Read the model definition and answer for the solid it produces. Units are mm, in the model's axes. Face numbers are marked on the shaded views. A direction names the side the tool comes from. Round coordinates to 2 decimals unless told otherwise and drop trailing zeros. Loops run counter-clockwise (first coordinate to the right, second up) from the corner with the lowest first, then second, coordinate; pieces in that order, holes last. Notation, with made-up numbers: M 52,84 L 72,84 A26 ccw 72,109 Z; hole C 48,37 d3. An arc over 180 degrees is marked long. Answer as CSV lines item,"result".
```python
from build123d import *

# Parameters (mm, degrees)
F0_W     = 48
F0_H     = 11
F1_DEPTH = 1.1
F0_W_2   = 52
F0_H_2   = 14
F2_DEPTH = 6
F3_R     = 0.925956
F4_DEPTH = 25


with BuildPart() as f1:
    # F0 (on Top) → F1 (new body)
    with BuildSketch(Plane.XY):
        Rectangle(F0_W, F0_H)
    extrude(amount=F1_DEPTH)

    # F0 (on Top) → F2 (join)
    with BuildSketch(Plane.XY):
        Rectangle(F0_W_2, F0_H_2)
        Rectangle(F0_W, F0_H, mode=Mode.SUBTRACT)
    extrude(amount=F2_DEPTH)

    # F3 (on face) → F4 (cut)
    with BuildSketch(Plane(origin=(24, 0, 0), x_dir=(0, -1, 0), z_dir=(-1, 0, 0))):
        with Locations((0, 3.55)):
            Circle(F3_R)
    extrude(amount=-F4_DEPTH, mode=Mode.SUBTRACT)


solid = f1.part
```
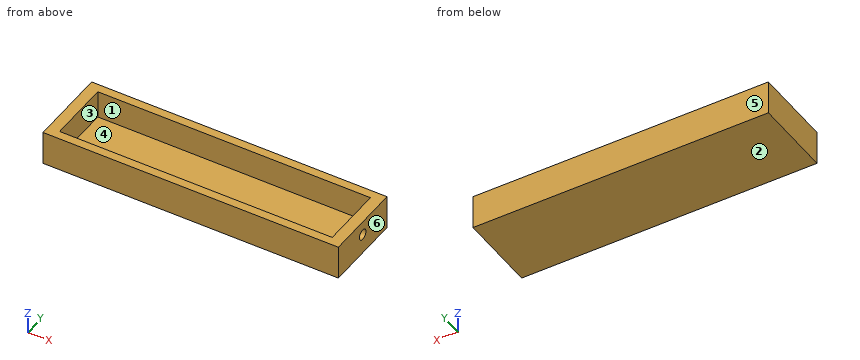
1) Find section D-D, the plane y = 0. Give the vertices of the cut face in (x, z).
Evaluation:
outline,"M -26,0 L 26,0 L 26,2.62 L 24,2.62 L 24,1.1 L -24,1.1 L -24,6 L -26,6 Z; M 24,4.48 L 26,4.48 L 26,6 L 24,6 Z"
2) Find section C-C, the plane x = 21. Give the vertices of the cut face in (y, z).
Evaluation:
outline,"M -7,0 L 7,0 L 7,6 L 5.5,6 L 5.5,1.1 L -5.5,1.1 L -5.5,6 L -7,6 Z"
3) This flat-tipped pin is pushed along its axis until it touches: P1, Ø5.5, axis at x = -11, y = 0.5, coming from the +Z side. Where does it stop, or does it pass through?
Evaluation:
P1,"stops at z = 1.1"
4) A tool of negligible diameter and unlimited length cuts with its end or side. For the marked faces 1 and 2, from which of +Z, -Z, +X, -X, +Y, -Y can it reach the whole face along a straight path? Write none if from no direction.
Evaluation:
face 1,"+Z"
face 2,"-Z, +X, -X, +Y, -Y"
5) Find section B-B, the plane z = 3.55. Give the vertices of the cut face in (x, y).
Evaluation:
outline,"M -26,-7 L 26,-7 L 26,-0.93 L 24,-0.93 L 24,-5.5 L -24,-5.5 L -24,5.5 L 24,5.5 L 24,0.93 L 26,0.93 L 26,7 L -26,7 Z"
6) Straight lines are drawn through the part: line 1 (Y direction, x = 4, z = 1.95); line 2 (Z direction, x = 25.55, y = 0); line 3 (X direction, y = 2.25, z = 5.75). For each, find the intervals that lie inside material, in ascending order.
Evaluation:
line 1,"y = -7 to -5.5, 5.5 to 7"
line 2,"z = 0 to 2.62, 4.48 to 6"
line 3,"x = -26 to -24, 24 to 26"
7) Determine the mould class of the marked faces 3, 4, 5 and 6 for opening direction Y: released by +Y, released by -Y, zero draft, split by the parting line, or undercut.
Evaluation:
face 3,"undercut"
face 4,"undercut"
face 5,"released by +Y"
face 6,"zero draft"
8) Find section A-A, the plane y = 2.5. Give the vertices of the cut face in (x, z), then the cut area to 3 significant figures.
Evaluation:
outline,"M -26,0 L 26,0 L 26,6 L 24,6 L 24,1.1 L -24,1.1 L -24,6 L -26,6 Z"
area,"76.8 mm^2"
